For this review, take the finished solid that the model builds, in its own axes (mm). A direction names the side the tool comes from. Round coordinates to 2 decimals unless told otherwise and drop trailing zeros. Order: outer loops, then holes, each group sorted by start corner. A loop starts at its lowest first (then second) coordinate and runs counter-clockwise, first axis right, second up.
from build123d import *

# Parameters (mm, degrees)
F0_W     = 40
F0_H     = 12
F0_R     = 6
F1_DEPTH = 16
F2_DEPTH = 24
F3_DEPTH = 64
F5_DEPTH = 100.001
F6_R     = 6.5
F7_DEPTH = 45.001


with BuildPart() as f1:
    # F0 (on Top) → F1 (new body)
    with BuildSketch(Plane.XY):
        with BuildLine():
            Line((50, 20), (50, 25))
            Line((50, 25), (-44, 25))
            ThreePointArc((-44, 25), (-48.2426406871, 23.2426406871), (-50, 19))
            Line((-50, 19), (-50, -19))
            ThreePointArc((-50, -19), (-48.2426406871, -23.2426406871), (-44, -25))
            Line((-44, -25), (50, -25))
            Line((50, -25), (50, -20))
            Line((50, -20), (10, -20))
            Line((10, -20), (-15, -20))
            ThreePointArc((-15, -20), (-35, 0), (-15, 20))
            Line((-15, 20), (10, 20))
            Line((10, 20), (50, 20))
        make_face()
        with Locations((30, 14)):
            Rectangle(F0_W, F0_H)
        with BuildLine():
            Line((10, 8), (10, 20))
            Line((10, 20), (-15, 20))
            ThreePointArc((-15, 20), (-35, 0), (-15, -20))
            Line((-15, -20), (10, -20))
            Line((10, -20), (10, -8))
            Line((10, -8), (5, -8))
            Line((5, -8), (5, 8))
            Line((5, 8), (10, 8))
        make_face()
        with Locations((-15, 0)):
            Circle(F0_R, mode=Mode.SUBTRACT)
        with Locations((30, -14)):
            Rectangle(F0_W, F0_H)
    extrude(amount=F1_DEPTH)

    # F0 (on Top) → F2 (join)
    with BuildSketch(Plane.XY):
        with BuildLine():
            Line((10, 8), (10, 20))
            Line((10, 20), (-15, 20))
            ThreePointArc((-15, 20), (-35, 0), (-15, -20))
            Line((-15, -20), (10, -20))
            Line((10, -20), (10, -8))
            Line((10, -8), (5, -8))
            Line((5, -8), (5, 8))
            Line((5, 8), (10, 8))
        make_face()
        with Locations((-15, 0)):
            Circle(F0_R, mode=Mode.SUBTRACT)
        with Locations((30, -14)):
            Rectangle(F0_W, F0_H)
        with Locations((30, 14)):
            Rectangle(F0_W, F0_H)
    extrude(amount=F2_DEPTH)

    # F0 (on Top) → F3 (join)
    with BuildSketch(Plane.XY):
        with Locations((30, -14)):
            Rectangle(F0_W, F0_H)
        with Locations((30, 14)):
            Rectangle(F0_W, F0_H)
    extrude(amount=F3_DEPTH)

    # F4 (on face) → F5 (cut, through all)
    with BuildSketch(Plane(origin=(-50, 0, 0), x_dir=(0, -1, 0), z_dir=(-1, 0, 0))):
        with BuildLine():
            Line((-13, 0), (13, 0))
            ThreePointArc((13, 0), (11.8284271247, 2.8284271247), (9, 4))
            Line((9, 4), (-9, 4))
            ThreePointArc((-9, 4), (-11.8284271247, 2.8284271247), (-13, 0))
        make_face()
    extrude(amount=-F5_DEPTH, mode=Mode.SUBTRACT)

    # F6 (on face) → F7 (cut, through all)
    with BuildSketch(Plane.XZ.offset(20)):
        with Locations((30, 44)):
            Circle(F6_R)
        with BuildLine():
            Line((10, 64), (10, 44))
            ThreePointArc((10, 44), (15.8578643763, 58.1421356237), (30, 64))
            Line((30, 64), (10, 64))
        make_face()
        with BuildLine():
            Line((50, 64), (30, 64))
            ThreePointArc((30, 64), (44.1421356237, 58.1421356237), (50, 44))
            Line((50, 44), (50, 64))
        make_face()
    extrude(amount=-F7_DEPTH, mode=Mode.SUBTRACT)


solid = f1.part
(1) Add section D-D on x = 28.5. Give the boundary of the cut face in (y, z), plus the area to 3 significant figures.
(2) Clearance check with flat-ended pins moving along their axes: P1, Ø20, axis at x = -11.5, y = 2.5, coming from the -Z side; P2, Ø13.5, axis at x = 19, z = 28.5, coming from the +Y side; P3, Ø3, axis at x = -11, y = 3.5, coming from the +Z side; P4, Ø5, axis at y = 4, z = 48.5, coming from the +X side. State where each tip first meets the part, or that it passes through.
(3) Tool access review of faces 4 (the face through (-35, 0, 20)), 5 (the face through (-0.7, 11.797, 2.859)), 6 (the face through (25, 20, 34)), 7 (the face through (28, -8, 27)), 8 (the face through (10, 14, 34)): name each direction out of +Z, -Z, +X, -X, +Y, -Y from which nothing blocks a thin tool from reaching the whole face with its end or side.
(4) Draft analysis for pull direction Y (two halves, no side actions). For faces 1 (the face through (-0.7, -11.859, 2.797)), 2 (the face through (2, -25, 8)), 3 (the face through (-1, -19, 0)), state which applies: pulls with the +Y half, pulls with the -Y half, needs draft (parallel to the pull), parting line crosses it, or undercut.
(5) Add section B-B on y = 0. Give the boundary of the cut face in (x, z).
(6) Wall thickness on L1, parallel to Y at x = 19.5, z = 30.5; L2, parallel to Y at x = -15, z = 9; L3, parallel to Z at x = 30, y = 17: over which ranges is each line inside the solid? List them lowest first.
(7) Add section C-C on x = 12. Give the boundary of the cut face in (y, z), plus the area to 3 significant figures.
(8) Add section A-A on z = 28.5. Give the boundary of the cut face in (x, y), plus the area to 3 significant figures.
Here are the results:
1. outline: (-25, 0) - (-13, 0) arc R4 cw to (-9, 4) - (-8, 4) - (-8, 37.68) - (-20, 37.68) - (-20, 16) - (-25, 16) - close; (-20, 50.32) - (-8, 50.32) - (-8, 63.94) - (-20, 63.94) - close; (8, 4) - (9, 4) arc R4 cw to (13, 0) - (25, 0) - (25, 16) - (20, 16) - (20, 37.68) - (8, 37.68) - close; (8, 50.32) - (20, 50.32) - (20, 63.94) - (8, 63.94) - close
1. area: 1,360 mm2
2. P1: stops at z = 1.94
2. P2: stops at y = 20
2. P3: stops at z = 24
2. P4: passes through
3. face 4: +Z, -X
3. face 5: -Z, +X, -X
3. face 6: +Z, +X, -X, +Y
3. face 7: +Z, -Z, +X
3. face 8: +Z, -X, +Y, -Y
4. face 1: undercut
4. face 2: pulls with the -Y half
4. face 3: needs draft
5. outline: (-50, 4) - (-21, 4) - (-21, 24) - (-35, 24) - (-35, 16) - (-50, 16) - close; (-9, 4) - (5, 4) - (5, 24) - (-9, 24) - close
6. L1: y = -20 to -8, 8 to 20
6. L2: y = -25 to -6, 6 to 25
6. L3: z = 0 to 37.5, 50.5 to 64
7. outline: (-25, 0) - (-13, 0) arc R4 cw to (-9, 4) - (-8, 4) - (-8, 52.72) - (-20, 52.72) - (-20, 16) - (-25, 16) - close; (8, 4) - (9, 4) arc R4 cw to (13, 0) - (25, 0) - (25, 16) - (20, 16) - (20, 52.72) - (8, 52.72) - close
7. area: 1,390 mm2
8. outline: (10, -20) - (50, -20) - (50, -8) - (10, -8) - close; (10, 8) - (50, 8) - (50, 20) - (10, 20) - close
8. area: 960 mm2
